```python
from build123d import *

# Parameters (mm, degrees)
BOSS_EXTRU_1_DEPTH      = 3
ESQUISSE2_W             = 113.5
ESQUISSE2_H             = 3
ESQUISSE2_H_2           = 45
BOSS_EXTRU_2_DEPTH      = 3
ESQUISSE3_W             = 113.5
ESQUISSE3_H             = 18
BOSS_EXTRU_3_DEPTH      = 40
ENL_V_MAT_EXTRU_1_DEPTH = 132.114678423


with BuildPart() as part:
    # Esquisse1 → Boss.-Extru.1 (new body)
    with BuildSketch(Plane(origin=(0, 0, 0), x_dir=(1, 0, 0), z_dir=(0, 1, 0))):
        with BuildLine():
            Line((-46.879360142, 43.789213198), (-39.379360142, 43.789213198))
            Line((-39.379360142, 43.789213198), (-39.379360142, 47.789213198))
            Line((-39.379360142, 47.789213198), (-152.879360142, 47.789213198))
            Line((-152.879360142, 47.789213198), (-152.879360142, 43.789213198))
            Line((-152.879360142, 43.789213198), (-144.879360142, 43.789213198))
            ThreePointArc((-144.879360142, 43.789213198), (-142.879360142, 45.789213198), (-140.879360142, 43.789213198))
            Line((-140.879360142, 43.789213198), (-50.879360142, 43.789213198))
            ThreePointArc((-50.879360142, 43.789213198), (-48.879360142, 45.789213198), (-46.879360142, 43.789213198))
        make_face()
        with BuildLine():
            Line((-39.379360142, 33.789213198), (-39.379360142, 43.789213198))
            Line((-39.379360142, 43.789213198), (-46.879360142, 43.789213198))
            ThreePointArc((-46.879360142, 43.789213198), (-48.879360142, 41.789213198), (-50.879360142, 43.789213198))
            Line((-50.879360142, 43.789213198), (-140.879360142, 43.789213198))
            ThreePointArc((-140.879360142, 43.789213198), (-142.879360142, 41.789213198), (-144.879360142, 43.789213198))
            Line((-144.879360142, 43.789213198), (-152.879360142, 43.789213198))
            Line((-152.879360142, 43.789213198), (-152.879360142, 33.789213198))
            Line((-152.879360142, 33.789213198), (-39.379360142, 33.789213198))
        make_face()
    extrude(amount=BOSS_EXTRU_1_DEPTH)

    # Esquisse2 → Boss.-Extru.2 (add)
    with BuildSketch(Plane.XY.offset(-33.789213198)):
        with Locations((-96.129360142, 1.5)):
            Rectangle(ESQUISSE2_W, ESQUISSE2_H)
        with Locations((-96.129360142, -22.5)):
            Rectangle(ESQUISSE2_W, ESQUISSE2_H_2)
    extrude(amount=BOSS_EXTRU_2_DEPTH)

    # Esquisse3 → Boss.-Extru.3 (add)
    with BuildSketch(Plane.XY.offset(-30.789213198)):
        with Locations((-96.129360142, -9)):
            Rectangle(ESQUISSE3_W, ESQUISSE3_H)
    extrude(amount=BOSS_EXTRU_3_DEPTH)

    # Esquisse5 → Enlèv. mat.-Extru.1 (cut, through all)
    with BuildSketch(Plane.ZY.offset(152.879360142)):
        Polygon((-30.789213198, 0), (9.210786802, -15), (9.210786802, 0), align=None)
    extrude(amount=-ENL_V_MAT_EXTRU_1_DEPTH, mode=Mode.SUBTRACT)


solid = part.part
```
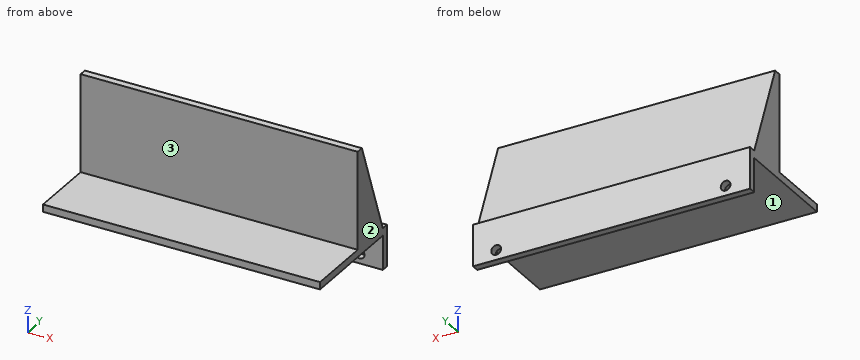
For this review, take the finished solid that the model builds, in its own axes (mm). Face numbers are marked on the shaded views. A direction names the side the tool comes from. Give positions to 0.01 mm unless a question says otherwise; leave off trailing zeros. Order: outer loops, then holes, each group sorted by start corner. A loop starts at its lowest first (then second) coordinate and runs counter-clockwise, first axis right, second up.
1) Take a section at D-D (z = -35). Give the boundary of the cut face in (x, y), then the cut area to 4 significant figures.
2) Wall thickness on line 1 (Z direction, x = -135, y = -29.5); line 2 (Y direction, x = -105, z = -39); line 3 (Z direction, x = -108, y = -17.5): over which ranges is each line inside the solid? List them lowest first.
3) Insertion check: pin 1 (1 mm diameter, centred on x = -55, z = -26.5, fed in from -Y); pin 2 (22.5 mm diameter, centred on x = -115.5, y = -12, fed in from -Z); pin 3 (1 mm diameter, centred on x = -106, y = -38, fed in from +Z); pin 4 (2.5 mm diameter, centred on x = -48.88, z = -43.79, fed in from +Y). Each pin has a flat end and moves straight along its axis. Give the tip position at first contact, or say it passes through.
4) Take a section at B-B (x = -143). Give the boundary of the cut face in (y, z).
5) Take a section at C-C (y = -27.5). Give the boundary of the cut face in (x, z), then the cut area to 4 significant figures.
6) For the marked faces 1, 2 and 3, list the 3-axis set-ups (+Z, -Z, +X, -X, +Y, -Y) from which the entire face can be reached by the end or side of a thin tool; tool diameter is ignored.
7) Take a section at A-A (x = -58.5). Give the boundary of the cut face in (y, z), then the cut area to 3 significant figures.
Derived:
1. outline: (-152.88, 0) - (-39.38, 0) - (-39.38, 3) - (-152.88, 3) - close
1. area: 340.5 mm2
2. line 1: z = -33.79 to -30.79
2. line 2: y = 0 to 3
2. line 3: z = -33.79 to 9.21
3. pin 1: stops at y = -18
3. pin 2: stops at z = -33.79
3. pin 3: stops at z = -30.79
3. pin 4: passes through
4. outline: (-45, -33.79) - (0, -33.79) - (0, -41.79) - (3, -41.79) - (3, -30.79) - (0, -30.79) - (-15, 9.21) - (-18, 9.21) - (-18, -30.79) - (-45, -30.79) - close; (0, -47.79) - (3, -47.79) - (3, -45.79) - (0, -45.79) - close
5. outline: (-152.88, -33.79) - (-39.38, -33.79) - (-39.38, -30.79) - (-152.88, -30.79) - close
5. area: 340.5 mm2
6. face 1: -Z, +X, -X, -Y
6. face 2: +Z, -Z, +X, +Y, -Y
6. face 3: +Z, +X, -X, -Y
7. outline: (-45, -33.79) - (0, -33.79) - (0, -47.79) - (3, -47.79) - (3, -30.79) - (0, -30.79) - (-15, 9.21) - (-18, 9.21) - (-18, -30.79) - (-45, -30.79) - close
7. area: 606 mm2
